The model under review builds one solid part; all positions refer to its coordinate system, in mm. A direction names the side the tool comes from. Round coordinates to 2 decimals unless told otherwise and drop trailing zeros. Write each loop counter-clockwise with the first axis right and the second up, starting at its lowest first coordinate (ties: lowest second). Pieces come first, ordered by that corner, then holes. Notation, with made-up numbers: (78, 86) -> (128, 86) arc R17 ccw to (128, 96) -> close; hole circle Ø6 at (64.25, 81). An arc over 180 degrees is marked (long way). Answer in a Markdown table with one row per item. Add a question column.
```python
from build123d import *

# Parameters (mm, degrees)
F4_R            = 3.5
F5_DEPTH        = 4
F6_D            = 2.5
F6_CBORE_D      = 4.5
F6_CBORE_DEPTH  = 2
F7_DEPTH        = 15
F9_D            = 3
F9_DEPTH        = 13.5
F9_CSINK_D      = 4
F9_CSINK_ANGLE  = 90
F9_TIP          = 0.9012909285
F11_D           = 3
F11_DEPTH       = 13.5
F11_CSINK_D     = 4
F11_CSINK_ANGLE = 90
F11_TIP         = 0.9012909285
F13_D           = 3
F13_DEPTH       = 13.5
F13_CSINK_D     = 4
F13_CSINK_ANGLE = 90
F13_TIP         = 0.9012909285
F15_D           = 3
F15_DEPTH       = 13.5
F15_CSINK_D     = 4
F15_CSINK_ANGLE = 90
F15_TIP         = 0.9012909285
F16_DEPTH       = 25
F18_DEPTH       = 4
F20_DEPTH       = 25
F21_DEPTH       = 25
F22_W           = 20
F22_H           = 30.4843550548
F22_H_2         = 31.25
F22_H_3         = 30.620081059
F23_DEPTH       = 4
F19_W           = 5
F19_H           = 5
F24_DEPTH       = 15


with BuildPart() as f5:
    # F4 (on Top) → F5 (new body)
    with BuildSketch(Plane.XY):
        Polygon((27.5709562153, 77.495081059), (-22.4290437847, 77.495081059), (-22.4290437847, 73.495081059), (-22.4290437847, -18.5049188996), (-22.4290437847, -22.504918941), (27.5709562153, -22.504918941), (27.5709562153, -18.504918941), (27.5709562153, 73.495081059), align=None)
        with BuildLine():
            ThreePointArc((-15.4290437847, -18.504918941), (-18.9290438054, -22.004918941), (-22.4290437847, -18.5049188996))
            ThreePointArc((-22.4290437847, -18.5049188996), (-18.9290437641, -15.004918941), (-15.4290437847, -18.504918941))
        make_face(mode=Mode.SUBTRACT)
        with Locations((24.0709562153, -18.504918941)):
            Circle(F4_R, mode=Mode.SUBTRACT)
        with BuildLine():
            ThreePointArc((-15.4290437847, 73.495081059), (-18.9290437847, 69.995081059), (-22.4290437847, 73.495081059))
            ThreePointArc((-22.4290437847, 73.495081059), (-18.9290437847, 76.995081059), (-15.4290437847, 73.495081059))
        make_face(mode=Mode.SUBTRACT)
        with Locations((24.0709562153, 73.495081059)):
            Circle(F4_R, mode=Mode.SUBTRACT)
        with BuildLine():
            ThreePointArc((-15.4290437847, -18.504918941), (-18.9290437641, -15.004918941), (-22.4290437847, -18.5049188996))
            ThreePointArc((-22.4290437847, -18.5049188996), (-18.9290438054, -22.004918941), (-15.4290437847, -18.504918941))
        make_face()
        with Locations((24.0709562153, -18.504918941)):
            Circle(F4_R)
        with BuildLine():
            ThreePointArc((-15.4290437847, 73.495081059), (-18.9290437847, 76.995081059), (-22.4290437847, 73.495081059))
            ThreePointArc((-22.4290437847, 73.495081059), (-18.9290437847, 69.995081059), (-15.4290437847, 73.495081059))
        make_face()
        with Locations((24.0709562153, 73.495081059)):
            Circle(F4_R)
    extrude(amount=F5_DEPTH)

    # F6 (through all)
    with Locations(Plane(origin=(0, 0, 0), x_dir=(1, 0, 0), z_dir=(0, 0, -1))):
        with Locations((19.5709562153, -69.995081059), (19.5709562153, 15.004918941), (-14.4290437847, 15.004918941), (-14.4290437847, -69.995081059)):
            CounterBoreHole(F6_D / 2, F6_CBORE_D / 2, F6_CBORE_DEPTH)

    # F4 (on Top) → F7 (join)
    with BuildSketch(Plane.XY):
        with BuildLine():
            ThreePointArc((-15.4290437847, -18.504918941), (-18.9290437641, -15.004918941), (-22.4290437847, -18.5049188996))
            ThreePointArc((-22.4290437847, -18.5049188996), (-18.9290438054, -22.004918941), (-15.4290437847, -18.504918941))
        make_face()
        with Locations((24.0709562153, -18.504918941)):
            Circle(F4_R)
        with BuildLine():
            ThreePointArc((-15.4290437847, 73.495081059), (-18.9290437847, 76.995081059), (-22.4290437847, 73.495081059))
            ThreePointArc((-22.4290437847, 73.495081059), (-18.9290437847, 69.995081059), (-15.4290437847, 73.495081059))
        make_face()
        with Locations((24.0709562153, 73.495081059)):
            Circle(F4_R)
    extrude(amount=-F7_DEPTH)

    # F9
    with Locations(Plane(origin=(0, 0, -15), x_dir=(1, 0, 0), z_dir=(0, 0, -1))):
        with Locations((-18.9290437847, -73.495081059)):
            CounterSinkHole(F9_D / 2, F9_CSINK_D / 2, depth=F9_DEPTH, counter_sink_angle=F9_CSINK_ANGLE)
            with Locations((0, 0, -(F9_DEPTH + F9_TIP / 2))):  # 118° drill point
                Cone(0, F9_D / 2, F9_TIP, mode=Mode.SUBTRACT)

    # F11
    with Locations(Plane(origin=(0, 0, -15), x_dir=(1, 0, 0), z_dir=(0, 0, -1))):
        with Locations((-18.9290437847, 18.504918941)):
            CounterSinkHole(F11_D / 2, F11_CSINK_D / 2, depth=F11_DEPTH, counter_sink_angle=F11_CSINK_ANGLE)
            with Locations((0, 0, -(F11_DEPTH + F11_TIP / 2))):  # 118° drill point
                Cone(0, F11_D / 2, F11_TIP, mode=Mode.SUBTRACT)

    # F13
    with Locations(Plane(origin=(0, 0, -15), x_dir=(1, 0, 0), z_dir=(0, 0, -1))):
        with Locations((24.0709562153, -73.495081059)):
            CounterSinkHole(F13_D / 2, F13_CSINK_D / 2, depth=F13_DEPTH, counter_sink_angle=F13_CSINK_ANGLE)
            with Locations((0, 0, -(F13_DEPTH + F13_TIP / 2))):  # 118° drill point
                Cone(0, F13_D / 2, F13_TIP, mode=Mode.SUBTRACT)

    # F15
    with Locations(Plane(origin=(0, 0, -15), x_dir=(1, 0, 0), z_dir=(0, 0, -1))):
        with Locations((24.0709562153, 18.504918941)):
            CounterSinkHole(F15_D / 2, F15_CSINK_D / 2, depth=F15_DEPTH, counter_sink_angle=F15_CSINK_ANGLE)
            with Locations((0, 0, -(F15_DEPTH + F15_TIP / 2))):  # 118° drill point
                Cone(0, F15_D / 2, F15_TIP, mode=Mode.SUBTRACT)

    # F16 (add): a face of the model
    f16_faces = [f5.faces().sort_by_distance(p)[0] for p in [
        (2.5709562153, -22.504918941, 2),
    ]]
    extrude(f16_faces, amount=F16_DEPTH)

    # F17 (on face) → F18 (cut)
    with BuildSketch(Plane.XY.offset(4)):
        Polygon((2.5709562153, -42.504918941), (22.5709562153, -42.504918941), (22.5709562153, -22.0463977089), (-17.4290437847, -22.0463977089), (-17.4290437847, -42.504918941), align=None)
        with BuildLine():
            Line((2.5709562153, -46.254918941), (2.5709562153, -43.754918941))
            ThreePointArc((2.5709562153, -43.754918941), (1.3209562153, -45.004918941), (2.5709562153, -46.254918941))
        make_face()
        with BuildLine():
            ThreePointArc((3.8209562153, -45.004918941), (3.4548396917, -44.1210354645), (2.5709562153, -43.754918941))
            Line((2.5709562153, -43.754918941), (2.5709562153, -46.254918941))
            ThreePointArc((2.5709562153, -46.254918941), (3.4548396917, -45.8888024175), (3.8209562153, -45.004918941))
        make_face()
    extrude(amount=-F18_DEPTH, mode=Mode.SUBTRACT)

    # F20 (add): a face of the model
    f20_faces = [f5.faces().sort_by_distance(p)[0] for p in [
        (27.5709562153, 14.995081059, 2),
    ]]
    extrude(f20_faces, amount=F20_DEPTH)

    # F21 (add): a face of the model
    f21_faces = [f5.faces().sort_by_distance(p)[0] for p in [
        (-22.4290437847, 14.995081059, 2),
    ]]
    extrude(f21_faces, amount=F21_DEPTH)

    # F22 (on face) → F23 (cut)
    with BuildSketch(Plane.XY.offset(4)):
        with Locations((-32.4290437847, -23.6845964684)):
            Rectangle(F22_W, F22_H)
        with Locations((-32.4290437847, 14.995081059)):
            Rectangle(F22_W, F22_H_2)
        with Locations((-32.4290437847, 54.057581059)):
            Rectangle(F22_W, F22_H_2)
        with Locations((37.5709562153, 54.057581059)):
            Rectangle(F22_W, F22_H_2)
        with Locations((37.5709562153, 15.3100405295)):
            Rectangle(F22_W, F22_H_3)
        with Locations((37.5709562153, -24.067418941)):
            Rectangle(F22_W, F22_H_2)
    extrude(amount=-F23_DEPTH, mode=Mode.SUBTRACT)

    # F19 (on face) → F24 (join)
    with BuildSketch(Plane(origin=(0, 0, 0), x_dir=(1, 0, 0), z_dir=(0, 0, -1))):
        with Locations((-19.9290437847, 45.004918941)):
            Rectangle(F19_W, F19_H)
        with Locations((25.0709562153, 45.004918941)):
            Rectangle(F19_W, F19_H)
    extrude(amount=F24_DEPTH)


solid = f5.part
```
1. Add section B-B on y = 14.5. Write out the cut boundary in (x, z).
2. Add section C-C on x = -26.5. Write out the cut boundary in (y, z), plus the area to 3 significant figures.
3. Add section D-D on z = -10.5. State how many separate pieces and enclosed holes the cut face has, plus the area to 3 significant figures.
4. Mouldability with a two-part tool opening along X and no side actions: class faces 1 (the flat face through (-33, -38.927, 2)), 2 (the flat face through (25, -45, -15)) as pulls with the +X half, pulls with the -X half, needs draft (parallel to the pull), parting line crosses it, or undercut.
5. Insertion check: pin 1 Ø2 at (x, y) = (19.57, 70) entering from -Z; pin 2 Ø5.5 at (x, y) = (-0.5, -46) entering from -Z; pin 3 Ø8 at (y, z) = (-16.5, -6) entering from +X; pin 4 Ø3 at (x, y) = (19.57, -15) entering from -Z. Each pin has a flat end and moves straight along its axis. Give the tip position at first contact, or say it passes through.
6. Tool access review of faces 3 (the flat face through (27.571, -24, 2)), 4 (the flat face through (22.571, -45, -7)), 5 (the cylindrical face through (27.41, 74.55, -7.4)): name each direction out of +Z, -Z, +X, -X, +Y, -Y from which nothing blocks a thin tool from reaching the whole face with its end or side.
7. For L1, parallel to Y at x = -39, z = 3; L2, parallel to X at y = 20.5, z = 2.25; L3, parallel to Y at x = -6, z = 0.75, list the stretches that pass through material, from the lowest coordinate up.
8. Add section A-A on x = 10. Write out the cut boundary in (y, z), plus the area to 3 significant figures.
Filled in:
| question | item | result |
|---|---|---|
| 1 | outline | (-47.43, 0) -> (-42.43, 0) -> (-42.43, 4) -> (-47.43, 4) -> close; (-22.43, 0) -> (27.57, 0) -> (27.57, 4) -> (-22.43, 4) -> close; (47.57, 0) -> (52.57, 0) -> (52.57, 4) -> (47.57, 4) -> close |
| 2 | outline | (-47.5, 0) -> (-38.93, 0) -> (-38.93, 4) -> (-47.5, 4) -> close; (-8.44, 0) -> (-0.63, 0) -> (-0.63, 4) -> (-8.44, 4) -> close; (30.62, 0) -> (38.43, 0) -> (38.43, 4) -> (30.62, 4) -> close; (69.68, 0) -> (77.5, 0) -> (77.5, 4) -> (69.68, 4) -> close |
| 2 | area | 128 mm² |
| 3 | separate pieces | 6 |
| 3 | enclosed holes | 4 |
| 3 | area | 176 mm² |
| 4 | face 1 | undercut |
| 4 | face 2 | needs draft |
| 5 | pin 1 | through |
| 5 | pin 2 | z = 0 |
| 5 | pin 3 | x = 27.57 |
| 5 | pin 4 | z = 2 |
| 6 | face 3 | +Z, -Z |
| 6 | face 4 | -Z, -Y |
| 6 | face 5 | -Z |
| 7 | L1 | -47.5 to -38.93, -8.44 to -0.63, 30.62 to 38.43, 69.68 to 77.5 |
| 7 | L2 | -47.43 to -42.43, -22.43 to 27.57, 47.57 to 52.57 |
| 7 | L3 | -47.5 to -42.5, -22.05 to 77.5 |
| 8 | outline | (-47.5, 0) -> (-42.5, 0) -> (-42.5, 4) -> (-47.5, 4) -> close; (-22.05, 0) -> (77.5, 0) -> (77.5, 4) -> (-22.05, 4) -> close |
| 8 | area | 418 mm² |
